```python
from build123d import *

# Parameters (mm, degrees)
BOSS_EXTRUDE1_DEPTH          = 64
SHELL1_T                     = -4
FILLET1_R                    = 10
FILLET2_R                    = 10
FILLET4_R                    = 10
FILLET6_R                    = 10
SKETCH3_W                    = 95
SKETCH3_H                    = 4
BOSS_EXTRUDE4_DEPTH          = 15
SKETCH4_W                    = 4
SKETCH4_H                    = 80
BOSS_EXTRUDE5_DEPTH          = 15
FILLET7_R                    = 5
FILLET8_R                    = 5
CSK_FOR_M3_SFHCS1_AT_2_COUNT = 2
CSK_FOR_M3_SFHCS1_AT_2_PITCH = 35
CSK_FOR_M3_SFHCS1_AT_3_COUNT = 2
CSK_FOR_M3_SFHCS1_AT_3_PITCH = 60
CSK_FOR_M3_SFHCS1_AT_4_COUNT = 2
CSK_FOR_M3_SFHCS1_AT_4_PITCH = 95
CSK_FOR_M3_SFHCS1_AT_5_COUNT = 2
CSK_FOR_M3_SFHCS1_AT_5_PITCH = 97.082439195
CSK_FOR_M3_SFHCS1_AT_6_COUNT = 2
CSK_FOR_M3_SFHCS1_AT_6_PITCH = 103.07764064
CSK_FOR_M3_SFHCS1_AT_7_COUNT = 2
CSK_FOR_M3_SFHCS1_AT_7_PITCH = 112.361025271


with BuildPart() as part:
    # Sketch1 → Boss-Extrude1 (new, symmetric)
    with BuildSketch(Plane.XY):
        Polygon((-47.5, -32.5), (47.5, -32.5), (47.5, 32.5), (-10, 32.5), (-10, 45.5), (-47.5, 45.5), (-47.5, 32.5), align=None)
    extrude(amount=BOSS_EXTRUDE1_DEPTH, both=True)

    # Shell1
    shell1_openings = [part.faces().sort_by_distance(p)[0] for p in [
        (0, -32.5, 0),
        (-47.5, 6.5, 0),
        (47.5, 0, 0),
    ]]
    offset(amount=SHELL1_T, openings=shell1_openings, kind=Kind.INTERSECTION)

    # Fillet1
    fillet1_edges = [part.edges().sort_by_distance(p)[0] for p in [
        (-10, 32.5, 0),
    ]]
    fillet(fillet1_edges, radius=FILLET1_R)

    # Fillet2
    fillet2_edges = [part.edges().sort_by_distance(p)[0] for p in [
        (-10, 45.5, 0),
    ]]
    fillet(fillet2_edges, radius=FILLET2_R)

    # Fillet4
    fillet4_edges = [part.edges().sort_by_distance(p)[0] for p in [
        (-14, 28.5, 0),
    ]]
    fillet(fillet4_edges, radius=FILLET4_R)

    # Fillet6
    fillet6_edges = [part.edges().sort_by_distance(p)[0] for p in [
        (-14, 41.5, 0),
    ]]
    fillet(fillet6_edges, radius=FILLET6_R)

    # Sketch3 → Boss-Extrude4 (add)
    with BuildSketch(Plane.XZ.offset(32.5)):
        with Locations((0, 62)):
            Rectangle(SKETCH3_W, SKETCH3_H)
        with Locations((0, -62)):
            Rectangle(SKETCH3_W, SKETCH3_H)
    extrude(amount=BOSS_EXTRUDE4_DEPTH)

    # Sketch4 → Boss-Extrude5 (add)
    with BuildSketch(Plane.ZY.offset(-47.5)):
        with Locations((62, -7.5)):
            Rectangle(SKETCH4_W, SKETCH4_H)
        with Locations((-62, -7.5)):
            Rectangle(SKETCH4_W, SKETCH4_H)
    extrude(amount=-BOSS_EXTRUDE5_DEPTH)

    # Fillet7
    fillet7_edges = [part.edges().sort_by_distance(p)[0] for p in [
        (21.75, 28.5, -60),
        (21.75, 28.5, 60),
        (-9.700877125, 30.284161637, -60),
        (-9.700877125, 30.284161637, 60),
        (-35.117496998, 41.5, -60),
        (-17.03411687, 39.715838363, -60),
        (-35.117496998, 41.5, 60),
        (-17.03411687, 39.715838363, 60),
    ]]
    fillet(fillet7_edges, radius=FILLET7_R)

    # Fillet8
    fillet8_edges = [part.edges().sort_by_distance(p)[0] for p in [
        (-5.700877125, 34.284161637, 64),
        (-33.117496998, 45.5, -64),
        (-33.117496998, 45.5, 64),
        (-5.700877125, 34.284161637, -64),
        (31.25, 32.5, 64),
        (31.25, 32.5, -64),
    ]]
    fillet(fillet8_edges, radius=FILLET8_R)

    # Sketch6 → CSK for M3 SFHCS1 (revolve, cut)
    with BuildSketch(Plane(origin=(-40, -40, -64), x_dir=(0, 1, 0), z_dir=(1, 0, 0))):
        Polygon((0, 0), (0, 16.021463052), (1.7, 15), (1.7, 1.66), (3.36, 0), align=None)
    csk_for_m3_sfhcs1 = revolve(axis=Axis((-40, -40, -70.35), (0, 0, 1)), mode=Mode.SUBTRACT)

    # CSK for M3 SFHCS1 at 2: CSK for M3 SFHCS1 ×2
    with Locations(*[(i * CSK_FOR_M3_SFHCS1_AT_2_PITCH, 0, 0) for i in range(1, CSK_FOR_M3_SFHCS1_AT_2_COUNT)]):
        add(csk_for_m3_sfhcs1, mode=Mode.SUBTRACT)

    # CSK for M3 SFHCS1 at 3: CSK for M3 SFHCS1 ×2
    with Locations(*[(i * CSK_FOR_M3_SFHCS1_AT_3_PITCH, 0, 0) for i in range(1, CSK_FOR_M3_SFHCS1_AT_3_COUNT)]):
        add(csk_for_m3_sfhcs1, mode=Mode.SUBTRACT)

    # CSK for M3 SFHCS1 at 4: CSK for M3 SFHCS1 ×2
    with Locations(*[(i * CSK_FOR_M3_SFHCS1_AT_4_PITCH, 0, 0) for i in range(1, CSK_FOR_M3_SFHCS1_AT_4_COUNT)]):
        add(csk_for_m3_sfhcs1, mode=Mode.SUBTRACT)

    # CSK for M3 SFHCS1 at 5: CSK for M3 SFHCS1 ×2
    with Locations(*[Vector(0.978549784986749, 0.2060104810498419, 0) * (i * CSK_FOR_M3_SFHCS1_AT_5_PITCH) for i in range(1, CSK_FOR_M3_SFHCS1_AT_5_COUNT)]):
        add(csk_for_m3_sfhcs1, mode=Mode.SUBTRACT)

    # CSK for M3 SFHCS1 at 6: CSK for M3 SFHCS1 ×2
    with Locations(*[Vector(0.9216353751380653, 0.3880570000581328, 0) * (i * CSK_FOR_M3_SFHCS1_AT_6_PITCH) for i in range(1, CSK_FOR_M3_SFHCS1_AT_6_COUNT)]):
        add(csk_for_m3_sfhcs1, mode=Mode.SUBTRACT)

    # CSK for M3 SFHCS1 at 7: CSK for M3 SFHCS1 ×2
    with Locations(*[Vector(0.8454889030309711, 0.5339929913879818, 0) * (i * CSK_FOR_M3_SFHCS1_AT_7_PITCH) for i in range(1, CSK_FOR_M3_SFHCS1_AT_7_COUNT)]):
        add(csk_for_m3_sfhcs1, mode=Mode.SUBTRACT)

    # Mirror1: CSK for M3 SFHCS1 across plane
    add(csk_for_m3_sfhcs1.mirror(Plane.XY), mode=Mode.SUBTRACT)

    # Mirror1 copy 1 sketch → Mirror1 copy 1 (revolve, cut)
    with BuildSketch(Plane(origin=(-5, -40, 64), x_dir=(0, 1, 0), z_dir=(1, 0, 0))):
        Polygon((0, 0), (0, -16.021463052), (1.7, -15), (1.7, -1.66), (3.36, 0), align=None)
    revolve(axis=Axis((-5, -40, 70.35), (0, 0, 1)), mode=Mode.SUBTRACT)

    # Mirror1 copy 2 sketch → Mirror1 copy 2 (revolve, cut)
    with BuildSketch(Plane(origin=(20, -40, 64), x_dir=(0, 1, 0), z_dir=(1, 0, 0))):
        Polygon((0, 0), (0, -16.021463052), (1.7, -15), (1.7, -1.66), (3.36, 0), align=None)
    revolve(axis=Axis((20, -40, 70.35), (0, 0, 1)), mode=Mode.SUBTRACT)

    # Mirror1 copy 3 sketch → Mirror1 copy 3 (revolve, cut)
    with BuildSketch(Plane(origin=(55, -40, 64), x_dir=(0, 1, 0), z_dir=(1, 0, 0))):
        Polygon((0, 0), (0, -16.021463052), (1.7, -15), (1.7, -1.66), (3.36, 0), align=None)
    revolve(axis=Axis((55, -40, 70.35), (0, 0, 1)), mode=Mode.SUBTRACT)

    # Mirror1 copy 4 sketch → Mirror1 copy 4 (revolve, cut)
    with BuildSketch(Plane(origin=(55, -20, 64), x_dir=(0, 1, 0), z_dir=(1, 0, 0))):
        Polygon((0, 0), (0, -16.021463052), (1.7, -15), (1.7, -1.66), (3.36, 0), align=None)
    revolve(axis=Axis((55, -20, 70.35), (0, 0, 1)), mode=Mode.SUBTRACT)

    # Mirror1 copy 5 sketch → Mirror1 copy 5 (revolve, cut)
    with BuildSketch(Plane(origin=(55, 0, 64), x_dir=(0, 1, 0), z_dir=(1, 0, 0))):
        Polygon((0, 0), (0, -16.021463052), (1.7, -15), (1.7, -1.66), (3.36, 0), align=None)
    revolve(axis=Axis((55, 0, 70.35), (0, 0, 1)), mode=Mode.SUBTRACT)

    # Mirror1 copy 6 sketch → Mirror1 copy 6 (revolve, cut)
    with BuildSketch(Plane(origin=(55, 20, 64), x_dir=(0, 1, 0), z_dir=(1, 0, 0))):
        Polygon((0, 0), (0, -16.021463052), (1.7, -15), (1.7, -1.66), (3.36, 0), align=None)
    revolve(axis=Axis((55, 20, 70.35), (0, 0, 1)), mode=Mode.SUBTRACT)


solid = part.part
```
Could you check a few things on this model? Use its own coordinates, in mm. A direction names the side the tool comes from. Give positions to 0.01 mm unless a question says otherwise; leave off trailing zeros. Loops run counter-clockwise (first coordinate to the right, second up) from the corner with the lowest first, then second, coordinate; pieces in that order, holes last. Notation, with made-up numbers: (27, 49) - (70, 49) arc R21 cw to (70, 66) - close; hole circle Ø7 at (69.5, 27). An arc over 180 degrees is marked (long way). Use one line per item in the form item = value.
1. I want a section at C-C (x = 32). Please give me the cut outline in (y, z), and give its area (3 significant figures).
Response values:
outline = (-47.5, -64) - (27.5, -64) arc R5 ccw to (32.5, -59) - (32.5, 59) arc R5 ccw to (27.5, 64) - (-47.5, 64) - (-47.5, 60) - (23.5, 60) arc R5 cw to (28.5, 55) - (28.5, -55) arc R5 cw to (23.5, -60) - (-47.5, -60) - close
area = 1,120 mm²
2. I need wall thicknesses on probe 1 along X at (y, z) = (-40, -61.2); probe 2 along Z at (x, y) = (-34.5, -18.5); probe 3 along X at (y, z) = (20, -61). Which ranges of each line are inside material? Lowest first, please.
Response values:
probe_1 = -47.5 to -41.7, -38.3 to -6.7, -3.3 to 18.3, 21.7 to 53.3, 56.7 to 62.5
probe_2 = -64 to -60, 60 to 64
probe_3 = -47.5 to 53.3, 56.7 to 62.5
3. I'm going to push flat-ended pins straight in: pin 1 Ø1.5 at (y, z) = (29.5, -5) entering from +X; pin 2 Ø4 at (x, y) = (55, 20) entering from -Z; pin 3 Ø5.5 at (x, y) = (20, -40) entering from -Z. Where does each tip first touch, or does it pass through?
Response values:
pin_1 = 47.5
pin_2 = -62.64
pin_3 = -63.39
4. Thinking about a two-plate mould opening in Y: for faces 4 (the face through (62.5, -7, 62)), 5 (the face through (53.85, -1.25, 61.19)), 6 (the face through (-32.92, 44, 62.57)), which applies, released by +Y, released by -Y, zero draft, split by the parting line, or undercut?
Response values:
face_4 = zero draft
face_5 = undercut
face_6 = released by +Y
5. On a 3-axis mill with a long thin cutter (end or side, diameter ignored), from which of +Z, -Z, +X, -X, +Y, -Y can I reach the whole of each face in a straight line? I mean faces 1 (the face through (23, 32.5, -1)), 2 (the face through (22, 28.5, 1)), 3 (the face through (54.49, 21.62, 61.19)). Say none if no direction works.
Response values:
face_1 = +Z, -Z, +X, +Y
face_2 = +X, -X, -Y
face_3 = +Z, -Z
6. I want a section at A-A (y = -26). Please give me the cut outline in (x, z).
Response values:
outline = (-47.5, -64) - (62.5, -64) - (62.5, -60) - (-47.5, -60) - close; (-47.5, 60) - (62.5, 60) - (62.5, 64) - (-47.5, 64) - close
7. I want a section at B-B (x = -40). Please give me the cut outline in (y, z), and give its area (3 significant figures).
Response values:
outline = (-47.5, -64) - (-43.36, -64) - (-41.7, -62.34) - (-41.7, -60) - (-47.5, -60) - close; (-47.5, 60) - (-41.7, 60) - (-41.7, 62.34) - (-43.36, 64) - (-47.5, 64) - close; (-38.3, -62.34) - (-36.64, -64) - (40.5, -64) arc R5 ccw to (45.5, -59) - (45.5, 59) arc R5 ccw to (40.5, 64) - (-36.64, 64) - (-38.3, 62.34) - (-38.3, 60) - (36.5, 60) arc R5 cw to (41.5, 55) - (41.5, -55) arc R5 cw to (36.5, -60) - (-38.3, -60) - close
area = 1,190 mm²
8. I want a section at D-D (x = 55). Give the number of separate pieces and of enclosed holes in the cut face, and give its area (3 significant figures).
Response values:
separate_pieces = 10
enclosed_holes = 0
area = 498 mm²
